Read the model definition and answer for the solid it produces. Units are mm, in the model's axes. A direction names the side the tool comes from. Coordinates: 2 decimals unless noted, no trailing zeros. Loops run counter-clockwise (first coordinate to the right, second up) from the corner with the lowest first, then second, coordinate; pieces in that order, holes last.
from build123d import *

# Parameters (mm, degrees)
SKETCH_1_R        = 50
EXTRUDE_1_DEPTH   = 50
SHELL_START       = 5
SHELL_1_OUTLINE_R = 40
SHELL_1_DEPTH     = 35
SKETCH_2_R        = 5
EXTRUDE_2_DEPTH   = 9


# Read off the part's stored shape, not the designer's step: 抽壳1
with BuildPart() as part:
    # 草图1 → 凸台-拉伸1 (new body)
    with BuildSketch(Plane(origin=(0, 0, 0), x_dir=(1, 0, 0), z_dir=(0, 1, 0))):
        with Locations(Location((0, 0, 0), (0, 0, 270))):
            Circle(SKETCH_1_R)
    extrude(amount=EXTRUDE_1_DEPTH)

    # 抽壳1 outline → 抽壳1 (cut)
    with BuildSketch(Plane(origin=(0, 0, 0), x_dir=(1, 0, 0), z_dir=(0, 1, 0)).offset(SHELL_START)):
        Circle(SHELL_1_OUTLINE_R)
    extrude(amount=SHELL_1_DEPTH, mode=Mode.SUBTRACT)

    # 草图2 → 凸台-拉伸2 (add)
    with BuildSketch(Plane.XZ):
        with Locations(Location((0, 0, 0), (0, 0, 90))):
            Circle(SKETCH_2_R)
    extrude(amount=EXTRUDE_2_DEPTH)


solid = part.part
Q1. A cutting plane is placed at A-A (x = 0). Give the vertices of the cut face in (y, z).
Findings below:
outline: (-9, -5) - (0, -5) - (0, -50) - (50, -50) - (50, 50) - (0, 50) - (0, 5) - (-9, 5) - close; hole (5, -40) - (40, -40) - (40, 40) - (5, 40) - close
Q2. A cutting plane is placed at C-C (y = 30). Give the vertices of the cut face in (x, z).
Findings below:
outline: circle Ø100 at (0, 0); hole circle Ø80 at (0, 0)
Q3. A cutting plane is placed at D-D (x = -32.5). Give the vertices of the cut face in (y, z).
Findings below:
outline: (0, -38) - (50, -38) - (50, 38) - (0, 38) - close; hole (5, -23.32) - (40, -23.32) - (40, 23.32) - (5, 23.32) - close
Q4. Flat-ended cylindrical pins translate along their axes: pin 1 Ø10 at (x, y) = (22.5, 43) entering from -Z; pin 2 Ø2 at (x, y) = (-25, 41) entering from -Z; pin 3 Ø10 at (x, z) = (-10, -1) entering from -Y; pin 4 Ø3 at (y, z) = (-2.5, 12) entering from -X (1 decimal). Find the tip coordinate at first contact, or state that the pin passes through.
Findings below:
pin 1: stops at z = -46.84
pin 2: stops at z = -43.86
pin 3: stops at y = 0
pin 4: passes through
Q5. Which of the six approach directions +Z, -Z, +X, -X, +Y, -Y give full straight-line access (tool end or side, diameter ignored) to faces 4 (the face through (-8.67, 22.26, 39.05)), 5 (the face through (0, -9, 0))?
Findings below:
face 4: none
face 5: +Z, -Z, +X, -X, -Y
Q6. Determine the mould class of faces 1 (the face through (-1, 40, -1)), 2 (the face through (1, 50, -1)), 3 (the face through (4.88, -4.44, -1.08)) for opening direction Z: +Z half, -Z half, draft (parallel to the pull), parting line (faces both ways), or undercut.
Findings below:
face 1: undercut
face 2: draft
face 3: parting line
Q7. A cutting plane is placed at B-B (z = 0). Give the vertices of the cut face in (x, y).
Findings below:
outline: (-50, 0) - (-5, 0) - (-5, -9) - (5, -9) - (5, 0) - (50, 0) - (50, 50) - (-50, 50) - close; hole (-40, 5) - (40, 5) - (40, 40) - (-40, 40) - close
Q8. Straight lines are drawn through the part: probe 1 along X at (y, z) = (24, 0); probe 2 along Z at (x, y) = (-1.5, 20); probe 3 along Y at (x, z) = (-29, 5.5). For each, find the intervals that lie inside material, in ascending order.
Findings below:
probe 1: x = -50 to -40, 40 to 50
probe 2: z = -49.98 to -39.97, 39.97 to 49.98
probe 3: y = 0 to 5, 40 to 50
